from build123d import *

# Parameters (mm, degrees)
BOSS_EXTRU_1_DEPTH           = 30
BOSS_EXTRU_2_DEPTH           = 1
ENL_V_MAT_EXTRU_2_DEPTH      = 70.865943062
ENL_V_MAT_EXTRU_2_DEPTH_BACK = 3
ENL_V_MAT_EXTRU_3_DEPTH      = 70.865943062
ENL_V_MAT_EXTRU_3_DEPTH_BACK = 3
COQUE3_OUTLINE_R             = 7
COQUE3_DEPTH                 = 24
COQUE3_START                 = 24
COQUE3_2_OUTLINE_R           = 7
COQUE3_2_DEPTH               = 3
COQUE3_START_2               = 27
COQUE3_3_DEPTH               = 1
CONG_1_R                     = 0.5
CONG_2_R                     = 1.5


# Read off the part's stored shape, not the designer's step: Coque3
with BuildPart() as part:
    # Esquisse1 → Boss.-Extru.1 (new body)
    with BuildSketch(Plane.XY):
        with BuildLine():
            Line((-35, -35), (-6.614378278, -35))
            ThreePointArc((-6.614378278, -35), (0, -52.5), (6.614378278, -35))
            Line((6.614378278, -35), (35, -35))
            Line((35, -35), (35, 35))
            Line((35, 35), (6.614378278, 35))
            ThreePointArc((6.614378278, 35), (0, 17.5), (-6.614378278, 35))
            Line((-6.614378278, 35), (-35, 35))
            Line((-35, 35), (-35, -35))
        make_face()
    extrude(amount=BOSS_EXTRU_1_DEPTH)

    # Esquisse4 → Boss.-Extru.2 (add)
    with BuildSketch(Plane.XY.offset(30)):
        Polygon((0, -24.5), (-12, -12.5), (-2, -12.5), (-2, 9.5), (2, 9.5), (2, -12.5), (12, -12.5), align=None)
    extrude(amount=BOSS_EXTRU_2_DEPTH)

    # Esquisse5 → Enlèv. mat.-Extru.2 (cut, two sides: drawn at the far end of the back side and taken through both)
    with BuildSketch(Plane.XY.offset(30).offset(-ENL_V_MAT_EXTRU_2_DEPTH_BACK)):
        Polygon((20, 251.700266086), (20, 35), (20, -35), (20, -251.700266086), (453.400532172, -251.700266086), (453.400532172, 251.700266086), align=None)
    extrude(amount=ENL_V_MAT_EXTRU_2_DEPTH + ENL_V_MAT_EXTRU_2_DEPTH_BACK, mode=Mode.SUBTRACT)

    # Esquisse6 → Enlèv. mat.-Extru.3 (cut, two sides: drawn at the far end of the back side and taken through both)
    with BuildSketch(Plane.XY.offset(30).offset(-ENL_V_MAT_EXTRU_3_DEPTH_BACK)):
        Polygon((-20, 251.700266086), (-20, 35), (-20, -35), (-20, -251.700266086), (-453.400532172, -251.700266086), (-453.400532172, 251.700266086), align=None)
    extrude(amount=ENL_V_MAT_EXTRU_3_DEPTH + ENL_V_MAT_EXTRU_3_DEPTH_BACK, mode=Mode.SUBTRACT)

    # Coque3 outline → Coque3 (cut)
    with BuildSketch(Plane.XY):
        with Locations((0, -42.5)):
            Circle(COQUE3_OUTLINE_R)
        with BuildLine():
            Line((-32, -32), (32, -32))
            Line((32, -32), (32, 32))
            Line((32, 32), (12.196310918, 32))
            ThreePointArc((12.196310918, 32), (0, 14.5), (-12.196310918, 32))
            Line((-12.196310918, 32), (-32, 32))
            Line((-32, 32), (-32, -32))
        make_face()
    extrude(amount=COQUE3_DEPTH, mode=Mode.SUBTRACT)

    # Coque3 2 outline → Coque3 2 (cut)
    with BuildSketch(Plane.XY.offset(COQUE3_START)):
        with Locations((0, -42.5)):
            Circle(COQUE3_2_OUTLINE_R)
        with BuildLine():
            Line((-17, 32), (-17, -32))
            Line((-17, -32), (17, -32))
            Line((17, -32), (17, 32))
            Line((17, 32), (12.196310918, 32))
            ThreePointArc((12.196310918, 32), (0, 14.5), (-12.196310918, 32))
            Line((-12.196310918, 32), (-17, 32))
        make_face()
    extrude(amount=COQUE3_2_DEPTH, mode=Mode.SUBTRACT)

    # Coque3 3 outline → Coque3 3 (cut)
    with BuildSketch(Plane.XY.offset(COQUE3_START_2)):
        Polygon((4.757359313, -15.5), (-4.757359313, -15.5), (0, -20.257359313), align=None)
    extrude(amount=COQUE3_3_DEPTH, mode=Mode.SUBTRACT)

    # Congé1
    cong_1_edges = [part.edges().sort_by_distance(p)[0] for p in [
        (6.614378278, -35, 15),
        (-6.614378278, -35, 15),
    ]]
    fillet(cong_1_edges, radius=CONG_1_R)

    # Congé2
    cong_2_edges = [part.edges().sort_by_distance(p)[0] for p in [
        (-6.614378278, 35, 15),
        (6.614378278, 35, 15),
    ]]
    fillet(cong_2_edges, radius=CONG_2_R)


solid = part.part
CAD build for the part. Positions are in the model's coordinates, mm. A direction names the side the tool comes from. Coordinates: 2 decimals unless noted, no trailing zeros. Write each loop counter-clockwise with the first axis right and the second up, starting at its lowest first coordinate (ties: lowest second). Pieces come first, ordered by that corner, then holes. Notation, with made-up numbers: (51, 46.25) - (95, 46.25) arc R30 cw to (95, 73.25) - close; hole circle Ø1 at (8, 86.5). An arc over 180 degrees is marked (long way). Use a Markdown table: item, result. Add a question column.
Item 1: Band-saw the part on C-C, the plane z = 21. Give the cut face in (x, y), and give its area (3 significant figures).
Item 2: Band-saw the part on A-A, the plane y = 27.5. Give the cut face in (x, z), and give its area (3 significant figures).
Item 3: Mould opens along Y. For faces 1 (the face through (2, 17, 0)), 2 (the face through (0, -32, 13)), 3 (the face through (-5.9, -18.6, 30.5)) say: pulls with the +Y half, pulls with the -Y half, needs draft (parallel to the pull), parting line crosses it, or undercut.
Item 4: 3-axis set-ups, long thin cutter, end or side, ignore diameter. For faces 4 (the face through (6.1, -18.4, 30.5)), 5 (the face through (-32, 0, 12)), 6 (the face through (20, 0, 28)): which of +Z, -Z, +X, -X, +Y, -Y reach the whole face in a straight line?
Item 5: Band-saw the part on B-B, the plane x = -18. Give the cut face in (y, z).
Item 6: Drill centre lines: L1, parallel to X at y = 27.5, z = 8; L2, parallel to Y at x = -28.5, z = 5.5. Where is each one in solid material? Low to high. Write a range as from..to.
Item 7: Flat gauge pins, fed straight in: pin 1 (7.5 mm diameter, centred on x = 25, y = -13, fed in from +Z); pin 2 (2.5 mm diameter, centred on x = 0.5, y = -19, fed in from -Z); pin 3 (12 mm diameter, centred on x = -25.5, y = 8.5, fed in from +Z). Where does each tip first touch, or does it go through?
Item 8: Band-saw the part on D-D, the plane y = 4.5. Give the cut face in (x, z), and give its area (3 significant figures).
Numbers:
| question | item | result |
|---|---|---|
| 1 | outline | (-35, -35) - (-7.83, -35) arc R0.5 cw to (-7.45, -35.83) arc R10 ccw (long way) to (7.45, -35.83) arc R0.5 cw to (7.83, -35) - (35, -35) - (35, 35) - (9.81, 35) arc R1.5 ccw to (8.53, 32.72) arc R10 cw (long way) to (-8.53, 32.72) arc R1.5 ccw to (-9.81, 35) - (-35, 35) - close; hole (-32, -32) - (32, -32) - (32, 32) - (12.2, 32) arc R13 cw (long way) to (-12.2, 32) - (-32, 32) - close; hole circle Ø14 at (0, -42.5) |
| 1 | area | 1,030 mm2 |
| 2 | outline | (-35, 0) - (-32, 0) - (-32, 24) - (-17, 24) - (-17, 27) - (-13, 27) - (-13, 0) - (-10, 0) - (-10, 30) - (-20, 30) - (-20, 27) - (-35, 27) - close; (10, 0) - (13, 0) - (13, 27) - (17, 27) - (17, 24) - (32, 24) - (32, 0) - (35, 0) - (35, 27) - (20, 27) - (20, 30) - (10, 30) - close |
| 2 | area | 474 mm2 |
| 3 | face 1 | needs draft |
| 3 | face 2 | undercut |
| 3 | face 3 | pulls with the -Y half |
| 4 | face 4 | +Z, +X, -Y |
| 4 | face 5 | -Z |
| 4 | face 6 | +Z, +X, +Y, -Y |
| 5 | outline | (-35, 0) - (-32, 0) - (-32, 24) - (32, 24) - (32, 0) - (35, 0) - (35, 30) - (-35, 30) - close |
| 6 | L1 | -35..-32, -13..-10, 10..13, 32..35 |
| 6 | L2 | -35..-32, 32..35 |
| 7 | pin 1 | z = 27 |
| 7 | pin 2 | z = 27 |
| 7 | pin 3 | z = 30 |
| 8 | outline | (-35, 0) - (-32, 0) - (-32, 24) - (-17, 24) - (-17, 27) - (17, 27) - (17, 24) - (32, 24) - (32, 0) - (35, 0) - (35, 27) - (20, 27) - (20, 30) - (2, 30) - (2, 31) - (-2, 31) - (-2, 30) - (-20, 30) - (-20, 27) - (-35, 27) - close |
| 8 | area | 376 mm2 |
